```python
from build123d import *

# Parameters (mm, degrees)
SKETCH1_R           = 3.175
BOSS_EXTRUDE1_DEPTH = 6.35


with BuildPart() as part:
    # Sketch1 → Boss-Extrude1 (new body)
    with BuildSketch(Plane(origin=(0, 6.35, 0), x_dir=(1, 0, 0), z_dir=(0, 1, 0))):
        with BuildLine():
            Line((90.469806331, 44.117768919), (99.06, 44.117768919))
            ThreePointArc((99.06, 44.117768919), (100.856051224, 44.861717695), (101.6, 46.657768919))
            Line((101.6, 46.657768919), (101.6, 69.517768919))
            ThreePointArc((101.6, 69.517768919), (38.1, 133.017768919), (-25.4, 69.517768919))
            Line((-25.4, 69.517768919), (-25.4, -57.482231081))
            Line((-25.4, -57.482231081), (0, -57.482231081))
            Line((0, -57.482231081), (0, 69.517768919))
            ThreePointArc((0, 69.517768919), (37.814649281, 107.616700334), (76.19572572, 70.088454351))
            ThreePointArc((76.19572572, 70.088454351), (76.267828346, 69.524429509), (76.463595703, 68.990577514))
            Line((76.463595703, 68.990577514), (88.197961266, 45.521846387))
            ThreePointArc((88.197961266, 45.521846387), (89.134449307, 44.497115866), (90.469806331, 44.117768919))
        make_face()
        with Locations((64.743779314, 112.270663754)):
            Circle(SKETCH1_R, mode=Mode.SUBTRACT)
        with Locations((-12.7, 56.817768919)):
            Circle(SKETCH1_R, mode=Mode.SUBTRACT)
    extrude(amount=-BOSS_EXTRUDE1_DEPTH)


solid = part.part
```
Could you check a few things on this model? Use its own coordinates, in mm. A direction names the side the tool comes from. Give positions to 0.01 mm unless a question says otherwise; leave off trailing zeros. Loops run counter-clockwise (first coordinate to the right, second up) from the corner with the lowest first, then second, coordinate; pieces in that order, holes last. Notation, with made-up numbers: (-19, 53) -> (19, 53) arc R17 ccw to (19, 82) -> close; hole circle Ø3 at (-35.5, 24.25). An arc over 180 degrees is marked (long way). Put each result on its own line as item: value.
(1) Imagine slicing it at D-D on z = -20. Write out the boundary of the cut face in (x, y), plus the area to 3 significant figures.
Computed:
outline: (-25.4, 0) -> (0, 0) -> (0, 6.35) -> (-25.4, 6.35) -> close
area: 161 mm^2
(2) Imagine slicing it at B-B on z = -105. Write out the boundary of the cut face in (x, y), plus the area to 3 significant figures.
Computed:
outline: (-14.56, 0) -> (24.22, 0) -> (24.22, 6.35) -> (-14.56, 6.35) -> close; (51.98, 0) -> (90.76, 0) -> (90.76, 6.35) -> (51.98, 6.35) -> close
area: 493 mm^2
(3) For faces 5 (the face through (-11, 3.2, -59.5)), 6 (the face through (82.25, 3.22, -57.42)), which set-ups out of +Z, -Z, +X, -X, +Y, -Y let a thin tool reach every point of the face, with its end or its side?
Computed:
face 5: +Y, -Y
face 6: +Z, +Y, -Y
(4) Imagine slicing it at C-C on y = 3.5. State how many separate pieces and enclosed holes the cut face has, plus the area to 3 significant figures.
Computed:
separate pieces: 1
enclosed holes: 2
area: 7,700 mm^2
(5) I'm going to push a flat-ended pin straight in: pin 1 Ø2 at (x, y) = (26, 4) entering from -Z. Where does the tip first touch, or does it pass through?
Computed:
pin 1: z = -132.04
(6) Thinking about a two-plate mould opening in X: for faces 1 (the face through (95, 3, -44.118)), 2 (the face through (62.404, 3.219, -114.416)), 3 (the face through (39.496, 3.219, -133.002)), 4 (the face through (0, 3, -5)), which applies, pulls with the +X half, pulls with the -X half, needs draft (parallel to the pull), parting line crosses it, or undercut?
Computed:
face 1: needs draft
face 2: undercut
face 3: parting line crosses it
face 4: undercut
(7) Imagine slicing it at A-A on x = -12.7. Write out the boundary of the cut face in (y, z), plus the area to 3 significant figures.
Computed:
outline: (0, -107.62) -> (6.35, -107.62) -> (6.35, -59.99) -> (0, -59.99) -> close; (0, -53.64) -> (6.35, -53.64) -> (6.35, 57.48) -> (0, 57.48) -> close
area: 1,010 mm^2
(8) Please list where these lines run through material, in increasing order: probe 1 along Z at (x, y) = (-12.7, 2); probe 2 along X at (y, z) = (6, -77); probe 3 along X at (y, z) = (5.25, 50.5). Write a range as [from, to].
Computed:
probe 1: [-107.62, -59.99], [-53.64, 57.48]
probe 2: [-24.96, 0.74], [75.46, 101.16]
probe 3: [-25.4, 0]
